```python
from build123d import *

# Parameters (mm, degrees)
BOSS_EXTRUDE1_DEPTH = 640
BOSS_EXTRUDE2_DEPTH = 63
BOSS_EXTRUDE4_DEPTH = 7
SKETCH10_R          = 6
CUT_EXTRUDE3_DEPTH  = 7
FILLET5_R           = 5
SKETCH22_R          = 6
CUT_EXTRUDE4_DEPTH  = 335


with BuildPart() as part:
    # Sketch1 → Boss-Extrude1 (new body)
    with BuildSketch(Plane.XY):
        Polygon((0, 0), (0, 70), (70, 70), (70, 63), (7, 63), (7, 0), align=None)
    extrude(amount=BOSS_EXTRUDE1_DEPTH)

    # Sketch2 → Boss-Extrude2 (add)
    with BuildSketch(Plane(origin=(0, 0, 0), x_dir=(1, 0, 0), z_dir=(0, 1, 0))):
        Polygon((0, -640), (25, -683.301270189), (31.062177826, -679.801270189), (7, -640), align=None)
    extrude(amount=BOSS_EXTRUDE2_DEPTH)

    # Sketch9 → Boss-Extrude4 (add)
    with BuildSketch(Plane(origin=(0, 63, 0), x_dir=(1, 0, 0), z_dir=(0, 1, 0))):
        with BuildLine():
            Line((0, -640), (25, -683.301270189))
            ThreePointArc((25, -683.301270189), (29.250444511, -686.562750973), (34.562177826, -685.863448016))
            Line((34.562177826, -685.863448016), (70, -665.403411844))
            Line((70, -665.403411844), (70, -640))
            Line((70, -640), (0, -640))
        make_face()
    extrude(amount=BOSS_EXTRUDE4_DEPTH)

    # Sketch10 → Cut-Extrude3 (cut)
    with BuildSketch(Plane(origin=(-278.227615862, 0, 168.20474164), x_dir=(-0.5173609804017633, 0, -0.8557672674026079), z_dir=(0.8557672674026079, 0, -0.5173609804017633))):
        with Locations((-572.82203414, 35)):
            Circle(SKETCH10_R)
    extrude(amount=-CUT_EXTRUDE3_DEPTH, mode=Mode.SUBTRACT)

    # Fillet5
    fillet5_edges = [part.edges().sort_by_distance(p)[0] for p in [
        (7, 63, 320),
        (19.031088913, 63, 659.900635095),
    ]]
    fillet(fillet5_edges, radius=FILLET5_R)

    # Mirror6: part across plane


with BuildPart() as part_1:
    add(part.part)
    add(part.part.mirror(Plane.XY))

    # Sketch22 → Cut-Extrude4 (cut)
    with BuildSketch(Plane(origin=(0, 70, 0), x_dir=(1, 0, 0), z_dir=(0, 1, 0))):
        with Locations(Location((35, 0, 0), (0, 0, 270))):
            Circle(SKETCH22_R)
        with Locations(Location((35, 350, 0), (0, 0, 270))):
            Circle(SKETCH22_R)
        with Locations(Location((35, -500, 0), (0, 0, 270))):
            Circle(SKETCH22_R)
    extrude(amount=-CUT_EXTRUDE4_DEPTH, mode=Mode.SUBTRACT)


solid = part_1.part
```
Design review of the part built by this model. Coordinates are the model's own, in mm. A direction names the side the tool comes from. Coordinates: 2 decimals unless noted, no trailing zeros. Order: outer loops, then holes, each group sorted by start corner. A loop starts at its lowest first (then second) coordinate and runs counter-clockwise, first axis right, second up. Notation, with made-up numbers: (76.25, 67) -> (103.25, 67) arc R17 ccw to (103.25, 78) -> close; hole circle Ø2 at (20.5, 6.25). An arc over 180 degrees is marked (long way). One line per item, written item: value. Start each with the question number.
Q1. Tool access review of faces 4 (the flat face through (19.2, 28.59, 660.18)), 5 (the flat face through (12.325, 42.288, -661.348)): name each direction out of +Z, -Z, +X, -X, +Y, -Y from which nothing blocks a thin tool from reaching the whole face with its end or side.
Q2. For probe 1 along X at (y, z) = (66, -350); probe 2 along X at (y, z) = (33, 400); probe 3 along Y at (x, z) = (65, 506), list the stretches that pass through material, from the lowest coordinate up.
Q3. Mouldability with a two-part tool opening along Z and no side actions: class faces 1 (the flat face through (12.325, 42.288, 661.348)), 2 (the flat face through (35, 70, 10)), 3 (the cylindrical face through (20.109, 61.496, 658.927)) as pulls with the +Z half, pulls with the -Z half, needs draft (parallel to the pull), parting line crosses it, or undercut.
Q4. Take a section at A-A, the plane z = 34. State the section outline as (x, y) points.
Q5. Insertion check: pin 1 Ø8 at (x, y) = (11.5, 32) entering from -Z; pin 2 Ø1.5 at (x, y) = (27.5, 19) entering from +Z; pin 3 Ø2 at (y, z) = (58, 260) entering from -X; pin 4 Ø1.5 at (y, z) = (23.5, 261.5) entering from +X. Each pin has a flat end and moves straight along its axis. Give the tip position at first contact, or say it passes through.
Q6. Take a section at B-B, the plane x = 52.5. State the section outline as (y, z) points.
Values follow:
1. face 4: +X, -Y
1. face 5: -Z, -X, +Y, -Y
2. probe 1: x = 0 to 29, 41 to 70
2. probe 2: x = 0 to 7
2. probe 3: y = 63 to 70
3. face 1: pulls with the +Z half
3. face 2: needs draft
3. face 3: undercut
4. outline: (0, 0) -> (7, 0) -> (7, 58) arc R5 cw to (12, 63) -> (70, 63) -> (70, 70) -> (0, 70) -> close
5. pin 1: stops at z = -666.85
5. pin 2: stops at z = 682.29
5. pin 3: stops at x = 0
5. pin 4: stops at x = 7
6. outline: (63, -675.51) -> (70, -675.51) -> (70, 675.51) -> (63, 675.51) -> close
